Part model, mm, in its own coordinate system. A direction names the side the tool comes from. Coordinates: 2 decimals unless noted, no trailing zeros. Loops run counter-clockwise (first coordinate to the right, second up) from the corner with the lowest first, then second, coordinate; pieces in that order, holes last. Notation, with made-up numbers: (62.5, 5.25) - (88.5, 5.25) arc R35 ccw to (88.5, 42.25) - close; hole circle Ø2 at (12, 70). An arc over 180 degrees is marked (long way). Use a Markdown table: item, result. Add a question column.
1. Band-saw the part on A-A, the plane y = 0. Give the cut face in (x, z) (3 decimals).
2. Band-saw the part on D-D, the plane x = 35. Give the cut face in (y, z) (3 decimals), plus the area to 3 significant figures.
3. Band-saw the part on C-C, the plane z = -1.75. Give the cut face in (x, y).
4. Wall check: probe 1 along Y at (x, z) = (0, -6); probe 2 along Y at (x, z) = (0, 8.65); probe 3 along X at (y, z) = (-3, -2.25). Give the ranges that are in metal, low to high. Write a range as [from, to].
5. Drop flat-ended pins along their axis: pin 1 (4 mm diameter, centred on y = 30, z = 0, fed in from -X); pin 2 (8 mm diameter, centred on y = -7.5, z = 1, fed in from -X); pin 3 (2 mm diameter, centred on x = 14, z = 7, fed in from -Y). Give the stop position or say it passes through.
6. 3-axis set-ups, long thin cutter, end or side, ignore diameter. For faces 4 (the flat face through (22, 18, 6.35)), 5 (the flat face through (-20.4, -19.1, -9.525)): which of +Z, -Z, +X, -X, +Y, -Y reach the whole face in a straight line?
7. Pull direction Y, two halves, no side cores. Call faces 1 (the flat face through (9, -29, 9.525)), 2 (the cylindrical face through (42.397, 13.352, 0.133)), 3 (the cylindrical face through (-23.311, -17.874, 7.96)): pulls with the +Y half, pulls with the -Y half, needs draft (parallel to the pull), parting line crosses it, or undercut.
from build123d import *

# Parameters (mm, degrees)
F0_R     = 44.45
F1_DEPTH = 9.525
F2_R     = 29.3751
F3_DEPTH = 3.175
F4_R     = 27.7876
F5_DEPTH = 15.875


with BuildPart() as f1:
    # F0 (on Top) → F1 (new body, symmetric)
    with BuildSketch(Plane.XY):
        Circle(F0_R)
    extrude(amount=F1_DEPTH, both=True)

    # F2 (on face) → F3 (cut)
    with BuildSketch(Plane.XY.offset(9.525)):
        Circle(F2_R)
    extrude(amount=-F3_DEPTH, mode=Mode.SUBTRACT)

    # F4 (on face) → F5 (cut)
    with BuildSketch(Plane.XY.offset(6.35)):
        Circle(F4_R)
    extrude(amount=-F5_DEPTH, mode=Mode.SUBTRACT)


solid = f1.part
Geometry check:
| question | item | result |
|---|---|---|
| 1 | outline | (-44.45, -9.525) - (-27.788, -9.525) - (-27.788, 6.35) - (-29.375, 6.35) - (-29.375, 9.525) - (-44.45, 9.525) - close; (27.788, -9.525) - (44.45, -9.525) - (44.45, 9.525) - (29.375, 9.525) - (29.375, 6.35) - (27.788, 6.35) - close |
| 2 | outline | (-27.401, -9.525) - (27.401, -9.525) - (27.401, 9.525) - (-27.401, 9.525) - close |
| 2 | area | 1,040 mm^2 |
| 3 | outline | circle Ø88.9 at (0, 0); hole circle Ø55.58 at (0, 0) |
| 4 | probe 1 | y = [-44.45, -27.79], [27.79, 44.45] |
| 4 | probe 2 | y = [-44.45, -29.38], [29.38, 44.45] |
| 4 | probe 3 | x = [-44.35, -27.63], [27.63, 44.35] |
| 5 | pin 1 | stops at x = -34.52 |
| 5 | pin 2 | stops at x = -44.31 |
| 5 | pin 3 | stops at y = -42.51 |
| 6 | face 4 | +Z |
| 6 | face 5 | -Z, +X, -X, +Y, -Y |
| 7 | face 1 | needs draft |
| 7 | face 2 | parting line crosses it |
| 7 | face 3 | undercut |
